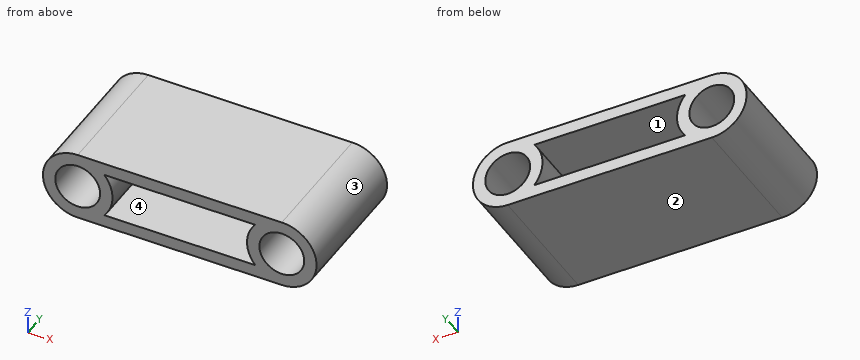
from build123d import *

# Parameters (mm, degrees)
F0_R     = 5.7546875
F1_DEPTH = 33.5359375


with BuildPart() as f1:
    # F0 (on Front) → F1 (new body)
    with BuildSketch(Plane.XZ):
        with BuildLine():
            Line((0, 8.9296875), (-52.3875, 8.9296875))
            ThreePointArc((-52.3875, 8.9296875), (-61.3171875, 0), (-52.3875, -8.9296875))
            Line((-52.3875, -8.9296875), (0, -8.9296875))
            ThreePointArc((0, -8.9296875), (8.9296875, 0), (0, 8.9296875))
        make_face()
        with Locations((-52.3875, 0)):
            Circle(F0_R, mode=Mode.SUBTRACT)
        with BuildLine():
            Line((-45.5594043193, 5.7546875), (-6.8280956807, 5.7546875))
            ThreePointArc((-6.8280956807, 5.7546875), (-8.9296875, 0), (-6.8280956807, -5.7546875))
            Line((-6.8280956807, -5.7546875), (-45.5594043193, -5.7546875))
            ThreePointArc((-45.5594043193, -5.7546875), (-43.4578125, 0), (-45.5594043193, 5.7546875))
        make_face(mode=Mode.SUBTRACT)
        Circle(F0_R, mode=Mode.SUBTRACT)
    extrude(amount=F1_DEPTH)


solid = f1.part
Can you work these out from the model? Positions are in its coordinate system, mm. Face numbers are marked on the shaded views. Coordinates: 2 decimals unless noted, no trailing zeros. Loops run counter-clockwise (first coordinate to the right, second up) from the corner with the lowest first, then second, coordinate; pieces in that order, holes last. Notation, with made-up numbers: (67, 66.5) - (122, 66.5) arc R17 cw to (122, 75.5) - close; hole circle Ø11 at (19.25, 62). An arc over 180 degrees is marked (long way). Answer as a JSON object with one key per item and string values. Group by question number.
Item 1: If we section it at B-B (y = -24): List the corners of the cut face in (x, z) for me, plus the area to 3 significant figures.
Item 2: If we section it at C-C (x = -39): List the corners of the cut face in (y, z) for me, plus the area to 3 significant figures.
Item 3: If we section it at A-A (z = 0): List the corners of the cut face in (x, y) for me, plus the area to 3 significant figures.
Item 4: If I drill on L1, parallel to Z at x = -35, y = -2; L2, parallel to X at y = -20.5, z = -3.75; L3, parallel to X at y = -18.5, z = -4.5, over which ranges is the centre line in solid material (lowest first)? Write a range as from..to.
Item 5: If we mould it in two halves opening along X, with no side actions, what happens to the marked faces 1, 2, 3 and 4? For each: released by +X, released by -X, zero draft, split by the parting line, or undercut.
Item 6: If we section it at D-D (x = 3): List the corners of the cut face in (y, z) for me, plus the area to 3 significant figures.
Item 7: For pin 1 (3 mm diameter, centred on y = -13.5, z = 5, fed in from -X); pin 2 (2 mm diameter, centred on y = -21, z = -5, fed in from -X); pin 3 (10.5 mm diameter, centred on x = 0, z = 0, fed in from +Y); pin 4 (2 mm diameter, centred on y = -15.5, z = 6, fed in from +X), each with a flat end and sliding along its axis, tell me the tip position at first contact or that it passes through.
Returned:
{
 "1": {"outline": "(-52.39, -8.93) - (0, -8.93) arc R8.93 ccw to (0, 8.93) - (-52.39, 8.93) arc R8.93 ccw to start; hole circle Ø11.51 at (-52.39, 0); hole (-45.56, -5.75) - (-6.83, -5.75) arc R8.93 cw to (-6.83, 5.75) - (-45.56, 5.75) arc R8.93 cw to start; hole circle Ø11.51 at (0, 0)", "area": "565 mm²"},
 "2": {"outline": "(-33.54, -8.93) - (0, -8.93) - (0, -5.75) - (-33.54, -5.75) - close; (-33.54, 5.75) - (0, 5.75) - (0, 8.93) - (-33.54, 8.93) - close", "area": "213 mm²"},
 "3": {"outline": "(-61.32, -33.54) - (-58.14, -33.54) - (-58.14, 0) - (-61.32, 0) - close; (-46.63, -33.54) - (-43.46, -33.54) - (-43.46, 0) - (-46.63, 0) - close; (-8.93, -33.54) - (-5.75, -33.54) - (-5.75, 0) - (-8.93, 0) - close; (5.75, -33.54) - (8.93, -33.54) - (8.93, 0) - (5.75, 0) - close", "area": "426 mm²"},
 "4": {"L1": "z = -8.93..-5.75, 5.75..8.93", "L2": "x = -60.49..-56.75, -48.02..-44.28, -8.1..-4.37, 4.37..8.1", "L3": "x = -60.1..-55.97, -48.8..-44.67, -7.71..-3.59, 3.59..7.71"},
 "5": {"face 1": "undercut", "face 2": "zero draft", "face 3": "released by +X", "face 4": "undercut"},
 "6": {"outline": "(-33.54, -8.41) - (0, -8.41) - (0, -4.91) - (-33.54, -4.91) - close; (-33.54, 4.91) - (0, 4.91) - (0, 8.41) - (-33.54, 8.41) - close", "area": "235 mm²"},
 "7": {"pin 1": "stops at x = -60.6", "pin 2": "stops at x = -60.37", "pin 3": "passes through", "pin 4": "stops at x = 7.4"}
}
